```python
from build123d import *

# Parameters (mm, degrees)
F0_W     = 1219.2
F0_H     = 609.6
F1_DEPTH = 304.8
F2_W     = 1168.4
F2_H     = 558.8
F3_DEPTH = 279.4
F3_TAPER = 20
F4_W     = 88.9
F4_H     = 88.9
F5_DEPTH = 609.6


with BuildPart() as f1:
    # F0 (on Front) → F1 (new body)
    with BuildSketch(Plane.XZ):
        with Locations((0, -90.1043365546)):
            Rectangle(F0_W, F0_H)
    extrude(amount=F1_DEPTH)

    # F2 (on face) → F3 (cut)
    with BuildSketch(Plane.XZ.offset(304.8)):
        with Locations((0, -90.1043365546)):
            Rectangle(F2_W, F2_H)
    extrude(amount=-F3_DEPTH, taper=F3_TAPER, mode=Mode.SUBTRACT)

    # F4 (on face) → F5 (join)
    with BuildSketch(Plane.XZ):
        with Locations((-565.15, -350.4543365546)):
            Rectangle(F4_W, F4_H)
        with Locations((565.15, -350.4543365546)):
            Rectangle(F4_W, F4_H)
        with Locations((565.15, 182.8677715369)):
            Rectangle(F4_W, F4_H)
        with Locations((-565.15, 182.8677715369)):
            Rectangle(F4_W, F4_H)
    extrude(amount=-F5_DEPTH)


solid = f1.part
```
Here's how the part is built. I have some questions about the finished solid (model axes, mm). A direction names the side the tool comes from. Round coordinates to 2 decimals unless told otherwise and drop trailing zeros. Loops run counter-clockwise (first coordinate to the right, second up) from the corner with the lowest first, then second, coordinate; pieces in that order, holes last.
1. Suppose I cut it at A-A, the plane y = 521.5. Please give me the cut outline in (x, z).
Answers:
outline: (-609.6, -394.9) - (-520.7, -394.9) - (-520.7, -306) - (-609.6, -306) - close; (-609.6, 138.42) - (-520.7, 138.42) - (-520.7, 227.32) - (-609.6, 227.32) - close; (520.7, -394.9) - (609.6, -394.9) - (609.6, -306) - (520.7, -306) - close; (520.7, 138.42) - (609.6, 138.42) - (609.6, 227.32) - (520.7, 227.32) - close
2. Thinking about a two-plate mould opening in X: for faces 6 (the face through (-5, -25.4, -97)), 7 (the face through (520.7, 301, -351)), 8 (the face through (-183, -304.8, 205)), 9 (the face through (609.6, -44, -88)), which applies, released by +X, released by -X, zero draft, split by the parting line, or undercut?
Answers:
face 6: undercut
face 7: undercut
face 8: zero draft
face 9: released by +X
3. For faces 1 (the face through (-9, -150, 214.696)), 2 (the face through (565, 301, 227.318)), 3 (the face through (-566, 301, -306.004)), 4 (the face through (-520.7, 301, 182)), 5 (the face through (-609.6, -57, -88)), which set-ups out of +Z, -Z, +X, -X, +Y, -Y let a thin tool reach every point of the face, with its end or its side?
Answers:
face 1: +Z, +X, -X, -Y
face 2: +Z, +X, -X, +Y, -Y
face 3: +X, -X, +Y
face 4: +Z, -Z, +Y
face 5: +Z, -Z, -X, +Y, -Y
4. If I drill on probe 1 along Z at (x, y) = (557.5, 350); probe 2 along Z at (x, y) = (445, -21.5); probe 3 along Y at (x, z) = (-89, -207), over which ranges is the centre line in solid material (lowest first)?
Answers:
probe 1: z = -394.9 to -306, 138.42 to 227.32
probe 2: z = -394.9 to 214.7
probe 3: y = -25.4 to 0
5. Will these pins go through, and if not, where does the flat tip stop? pin 1 (10 mm diameter, centred on x = 550.5, z = 219, fed in from -Y); pin 2 (4 mm diameter, centred on x = -147.5, z = -243.5, fed in from -Y); pin 3 (2 mm diameter, centred on x = 291, z = -266.5, fed in from +Y).
Answers:
pin 1: stops at y = -304.8
pin 2: stops at y = -25.4
pin 3: stops at y = 0
